```python
from build123d import *

# Parameters (mm, degrees)
SKETCH_1_R          = 2.5
SKETCH_1_R_2        = 1.75
SKETCH_1_W          = 20
SKETCH_1_H          = 10
EXTRUDE_1_DEPTH     = 4
SKETCH_2_W          = 39
SKETCH_2_H          = 39
CUT_EXTRUDE_1_DEPTH = 2.5
FILLET_1_R          = 3
FILLET_2_R          = 1
CHAMFER_1_SIZE      = 0.5
SKETCH_4_R          = 2.5
CUT_EXTRUDE_2_DEPTH = 2


with BuildPart() as part:
    # 草图1 → 凸台-拉伸1 (new body)
    with BuildSketch(Plane.XY):
        with BuildLine():
            Line((-103, -75), (103, -75))
            ThreePointArc((103, -75), (118.556349186, -68.556349186), (125, -53))
            Line((125, -53), (125, 53))
            ThreePointArc((125, 53), (118.556349186, 68.556349186), (103, 75))
            Line((103, 75), (-103, 75))
            ThreePointArc((-103, 75), (-118.556349186, 68.556349186), (-125, 53))
            Line((-125, 53), (-125, -53))
            ThreePointArc((-125, -53), (-118.556349186, -68.556349186), (-103, -75))
        make_face()
        with Locations((-114, 60)):
            Circle(SKETCH_1_R, mode=Mode.SUBTRACT)
        with Locations(Location((-114, -60, 0), (0, 0, 180))):
            Circle(SKETCH_1_R, mode=Mode.SUBTRACT)
        with Locations((-14, -60)):
            Circle(SKETCH_1_R, mode=Mode.SUBTRACT)
        with Locations(Location((-14, 60, 0), (0, 0, 180))):
            Circle(SKETCH_1_R, mode=Mode.SUBTRACT)
        with Locations((-85, 46)):
            Circle(SKETCH_1_R_2, mode=Mode.SUBTRACT)
        with Locations(Location((-25, 46, 0), (0, 0, 180))):
            Circle(SKETCH_1_R_2, mode=Mode.SUBTRACT)
        with Locations((-25, -46)):
            Circle(SKETCH_1_R_2, mode=Mode.SUBTRACT)
        with Locations(Location((-85, -46, 0), (0, 0, 180))):
            Circle(SKETCH_1_R_2, mode=Mode.SUBTRACT)
        with BuildLine():
            Line((-113, -40), (-107, -40))
            ThreePointArc((-107, -40), (-105.585786438, -39.414213562), (-105, -38))
            Line((-105, -38), (-105, 38))
            ThreePointArc((-105, 38), (-105.585786438, 39.414213562), (-107, 40))
            Line((-107, 40), (-113, 40))
            ThreePointArc((-113, 40), (-114.414213562, 39.414213562), (-115, 38))
            Line((-115, 38), (-115, -38))
            ThreePointArc((-115, -38), (-114.414213562, -39.414213562), (-113, -40))
        make_face(mode=Mode.SUBTRACT)
        with Locations((80, -24)):
            Rectangle(SKETCH_1_W, SKETCH_1_H, mode=Mode.SUBTRACT)
    extrude(amount=EXTRUDE_1_DEPTH)

    # 草图2 → 切除-拉伸1 (cut)
    with BuildSketch(Plane.XY.offset(4)):
        with Locations((80, 0)):
            Rectangle(SKETCH_2_W, SKETCH_2_H)
    extrude(amount=-CUT_EXTRUDE_1_DEPTH, mode=Mode.SUBTRACT)

    # 圆角1
    fillet_1_edges = [part.edges().sort_by_distance(p)[0] for p in [
        (90, -29, 2),
        (70, -29, 2),
    ]]
    fillet(fillet_1_edges, radius=FILLET_1_R)

    # 圆角2
    fillet_2_edges = [part.edges().sort_by_distance(p)[0] for p in [
        (70, -22.75, 4),
        (99.5, -19.5, 2.75),
        (99.5, 19.5, 2.75),
        (60.5, -19.5, 2.75),
        (60.5, 19.5, 2.75),
        (80, -29, 4),
        (90, -22.75, 4),
        (89.121320344, -28.121320344, 4),
        (70.878679656, -28.121320344, 4),
    ]]
    fillet(fillet_2_edges, radius=FILLET_2_R)

    # 倒角1
    chamfer_1_edges = [part.edges().sort_by_distance(p)[0] for p in [
        (90, -19.5, 2.25),
        (70, -19.5, 2.25),
        (99.5, 0, 4),
        (94.75, -19.5, 4),
        (65.25, -19.5, 4),
        (60.5, 0, 4),
        (80, 19.5, 4),
        (69.707106781, -19.5, 3.707106781),
        (90.292893219, -19.5, 3.707106781),
        (60.792893219, -19.207106781, 4),
        (99.207106781, -19.207106781, 4),
        (99.207106781, 19.207106781, 4),
        (60.792893219, 19.207106781, 4),
    ]]
    chamfer(chamfer_1_edges, length=CHAMFER_1_SIZE)

    # 草图4 → 切除-拉伸2 (cut)
    with BuildSketch(Plane.XY.offset(1.5)):
        with Locations((65.900290783, -14.099709217)):
            Circle(SKETCH_4_R)
        with Locations(Location((94.099709217, -14.099709217, 0), (0, 0, 180))):
            Circle(SKETCH_4_R)
        with Locations((94.099709217, 14.099709217)):
            Circle(SKETCH_4_R)
        with Locations(Location((65.900290783, 14.099709217, 0), (0, 0, 180))):
            Circle(SKETCH_4_R)
    extrude(amount=-CUT_EXTRUDE_2_DEPTH, mode=Mode.SUBTRACT)


solid = part.part
```
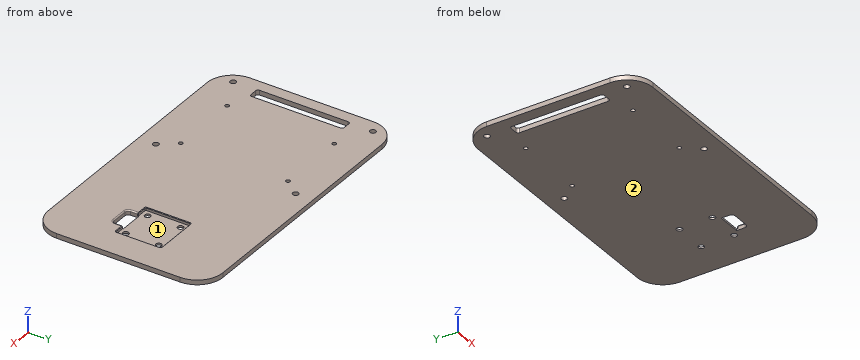
For this review, take the finished solid that the model builds, in its own axes (mm). Face numbers are marked on the shaded views. Round coordinates to 2 decimals unless told otherwise and drop trailing zeros. Loops run counter-clockwise (first coordinate to the right, second up) from the corner with the lowest first, then second, coordinate; pieces in that order, holes last.
Q1. To check wall thickness, follow line 1 along X through (y, z) = (15.5, 3.1); line 2 along Y through (x, z) = (-25, 0.9); line 3 along Y through (x, z) = (-114, 2.4). State the ranges of each line that lie inside material, in increasing order.
Result sheet:
line 1: x = -125 to -115, -105 to 60.5, 99.5 to 125
line 2: y = -75 to -47.75, -44.25 to 44.25, 47.75 to 75
line 3: y = -72.05 to -62.5, -57.5 to -39.73, 39.73 to 57.5, 62.5 to 72.05
Q2. Mouldability with a two-part tool opening along Y and no side actions: class the marked faces 1 and 2 as +Y half, -Y half, draft (parallel to the pull), parting line (faces both ways), or undercut.
Result sheet:
face 1: undercut
face 2: draft
Q3. Add section B-B on y = 32.5. Write out the cut boundary in (x, z), plus the area to 3 significant figures.
Result sheet:
outline: (-125, 0) - (-115, 0) - (-115, 4) - (-125, 4) - close; (-105, 0) - (125, 0) - (125, 4) - (-105, 4) - close
area: 960 mm2
Q4. Add section C-C on y = 60. Write out the cut boundary in (x, z).
Result sheet:
outline: (-123.86, 0) - (-116.5, 0) - (-116.5, 4) - (-123.86, 4) - close; (-111.5, 0) - (-16.5, 0) - (-16.5, 4) - (-111.5, 4) - close; (-11.5, 0) - (123.86, 0) - (123.86, 4) - (-11.5, 4) - close
Q5. Add section D-D on z = 2.2. Give the number of separate pieces and of enclosed holes in the cut face, plus the area to 3 significant figures.
Result sheet:
separate pieces: 1
enclosed holes: 10
area: 34,500 mm2
Q6. Add section A-A on x = -14. Write out the cut boundary in (y, z), plus the area to 3 significant figures.
Result sheet:
outline: (-75, 0) - (-62.5, 0) - (-62.5, 4) - (-75, 4) - close; (-57.5, 0) - (57.5, 0) - (57.5, 4) - (-57.5, 4) - close; (62.5, 0) - (75, 0) - (75, 4) - (62.5, 4) - close
area: 560 mm2
